Geometry check sheet. Reference: the model listing, model coordinates, mm. A direction names the side the tool comes from. Round coordinates to 2 decimals unless told otherwise and drop trailing zeros. Write each loop counter-clockwise with the first axis right and the second up, starting at its lowest first coordinate (ties: lowest second). Pieces come first, ordered by that corner, then holes. Notation, with made-up numbers: M 32,10 L 36,10 A22 ccw 36,41 Z; hole C 48,-11 d7. An arc over 180 degrees is marked long. One line per item, written item: value. Start each with the question number.
1. Section check C-C (x = 41). Record the boundary of the cut face in (y, z).
2. Depth check by flat-ended pin: P1, Ø5, axis at x = -25, z = -24, coming from the -Y side; P2, Ø1.5, axis at x = 97.5, z = 39.5, coming from the +Y side; P3, Ø0.6, axis at x = 139, z = 30, coming from the +Y side. Enter the tip coordinate at first touch or a pass-through.
3. Scan lines: probe 1 along Z at (x, y) = (125, -0.15); probe 2 along X at (y, z) = (8.5, 1); probe 3 along Z at (x, y) = (89, 10.25). Record each from-to range of solid material in increasing order. Write a range as [from, to].
4. Section check A-A (x = 125). Count the separate pieces of the cut face and the enclosed holes in it, and give its area (3 significant figures).
5. Access from +Z, -Z, +X, -X, +Y, -Y to the whole of each face (thin tool, end or side, straight path). Record for faces 1 (the cylindrical face through (120.786, -0.345, 0.553)), 2 (the flat face through (-71, 7, 71.3)), 3 (the flat face through (138.3, 6, 1)).
6. Release check for a two-part mould opening along X. For faces 4 (the flat face through (71, 7, -71.3)), 5 (the cylindrical face through (71.23, -0.35, 1.96)) record: pulls with the +X half, pulls with the -X half, needs draft (parallel to the pull), parting line crosses it, or undercut.
from build123d import *

# Parameters (mm, degrees)
SKETCH_1_W                         = 278
SKETCH_1_H                         = 144
SKETCH_1_R                         = 4.25
SM_BASE_FLANGE_1_DEPTH             = 0.7
SM_EDGE_FLANGE_1_STRIP_W           = 3.2
SM_EDGE_FLANGE_1_STRIP_H           = 0.7
SM_EDGE_FLANGE_1_STRIP_CUT_DEPTH   = 278
SM_EDGE_FLANGE_1_STRIP_2_W         = 3.2
SM_EDGE_FLANGE_1_STRIP_2_H         = 0.7
SM_EDGE_FLANGE_1_STRIP_CUT_2_DEPTH = 278
SM_EDGE_FLANGE_1_DEPTH             = 278
SM_EDGE_FLANGE_1_BEND_DEPTH        = 278
SKETCH_14_R                        = 3
CUT_EXTRUDE_1_DEPTH                = 10
SKETCH_15_R                        = 3
CUT_EXTRUDE_2_DEPTH                = 10
SKETCH_16_W                        = 3
SKETCH_16_H                        = 13.3
CUT_EXTRUDE_3_DEPTH                = 10
SKETCH_17_W                        = 3
SKETCH_17_H                        = 13.3
CUT_EXTRUDE_4_DEPTH                = 10
SM_EDGE_FLANGE_2_STRIP_W           = 3.2
SM_EDGE_FLANGE_2_STRIP_H           = 0.7
SM_EDGE_FLANGE_2_STRIP_CUT_DEPTH   = 142.2
SM_EDGE_FLANGE_2_STRIP_2_W         = 3.2
SM_EDGE_FLANGE_2_STRIP_2_H         = 0.7
SM_EDGE_FLANGE_2_STRIP_CUT_2_DEPTH = 142.2
SM_EDGE_FLANGE_2_DEPTH             = 142.2
SM_EDGE_FLANGE_2_BEND_DEPTH        = 142.2


# Sheet-metal steps are written as plain solids
with BuildPart() as part:
    # Sketch 1 → 基体-法兰1 (new body)
    with BuildSketch(Plane(origin=(0, 0, 0), x_dir=(1, 0, 0), z_dir=(0, 1, 0))):
        Rectangle(SKETCH_1_W, SKETCH_1_H)
        with Locations(Location((-125, -48, 0), (0, 0, 270))):
            Circle(SKETCH_1_R, mode=Mode.SUBTRACT)
        with Locations(Location((-125, -24, 0), (0, 0, 270))):
            Circle(SKETCH_1_R, mode=Mode.SUBTRACT)
        with Locations(Location((-125, 0, 0), (0, 0, 270))):
            Circle(SKETCH_1_R, mode=Mode.SUBTRACT)
        with Locations(Location((-125, 24, 0), (0, 0, 270))):
            Circle(SKETCH_1_R, mode=Mode.SUBTRACT)
        with Locations(Location((-125, 48, 0), (0, 0, 270))):
            Circle(SKETCH_1_R, mode=Mode.SUBTRACT)
        with Locations(Location((-75, -48, 0), (0, 0, 90))):
            Circle(SKETCH_1_R, mode=Mode.SUBTRACT)
        with Locations(Location((-75, -24, 0), (0, 0, 90))):
            Circle(SKETCH_1_R, mode=Mode.SUBTRACT)
        with Locations(Location((-75, 0, 0), (0, 0, 90))):
            Circle(SKETCH_1_R, mode=Mode.SUBTRACT)
        with Locations(Location((-75, 24, 0), (0, 0, 90))):
            Circle(SKETCH_1_R, mode=Mode.SUBTRACT)
        with Locations(Location((-75, 48, 0), (0, 0, 90))):
            Circle(SKETCH_1_R, mode=Mode.SUBTRACT)
        with Locations(Location((-25, -48, 0), (0, 0, 270))):
            Circle(SKETCH_1_R, mode=Mode.SUBTRACT)
        with Locations(Location((-25, -24, 0), (0, 0, 270))):
            Circle(SKETCH_1_R, mode=Mode.SUBTRACT)
        with Locations(Location((-25, 0, 0), (0, 0, 270))):
            Circle(SKETCH_1_R, mode=Mode.SUBTRACT)
        with Locations(Location((-25, 24, 0), (0, 0, 270))):
            Circle(SKETCH_1_R, mode=Mode.SUBTRACT)
        with Locations(Location((-25, 48, 0), (0, 0, 270))):
            Circle(SKETCH_1_R, mode=Mode.SUBTRACT)
        with Locations(Location((25, -48, 0), (0, 0, 90))):
            Circle(SKETCH_1_R, mode=Mode.SUBTRACT)
        with Locations(Location((25, -24, 0), (0, 0, 90))):
            Circle(SKETCH_1_R, mode=Mode.SUBTRACT)
        with Locations(Location((25, 0, 0), (0, 0, 90))):
            Circle(SKETCH_1_R, mode=Mode.SUBTRACT)
        with Locations(Location((25, 24, 0), (0, 0, 90))):
            Circle(SKETCH_1_R, mode=Mode.SUBTRACT)
        with Locations(Location((25, 48, 0), (0, 0, 90))):
            Circle(SKETCH_1_R, mode=Mode.SUBTRACT)
        with Locations(Location((75, 48, 0), (0, 0, 270))):
            Circle(SKETCH_1_R, mode=Mode.SUBTRACT)
        with Locations(Location((75, 24, 0), (0, 0, 270))):
            Circle(SKETCH_1_R, mode=Mode.SUBTRACT)
        with Locations(Location((75, 0, 0), (0, 0, 270))):
            Circle(SKETCH_1_R, mode=Mode.SUBTRACT)
        with Locations(Location((75, -24, 0), (0, 0, 270))):
            Circle(SKETCH_1_R, mode=Mode.SUBTRACT)
        with Locations(Location((75, -48, 0), (0, 0, 270))):
            Circle(SKETCH_1_R, mode=Mode.SUBTRACT)
        with Locations(Location((125, -48, 0), (0, 0, 90))):
            Circle(SKETCH_1_R, mode=Mode.SUBTRACT)
        with Locations(Location((125, -24, 0), (0, 0, 90))):
            Circle(SKETCH_1_R, mode=Mode.SUBTRACT)
        with Locations(Location((125, 0, 0), (0, 0, 90))):
            Circle(SKETCH_1_R, mode=Mode.SUBTRACT)
        with Locations(Location((125, 24, 0), (0, 0, 90))):
            Circle(SKETCH_1_R, mode=Mode.SUBTRACT)
        with Locations(Location((125, 48, 0), (0, 0, 90))):
            Circle(SKETCH_1_R, mode=Mode.SUBTRACT)
    extrude(amount=-SM_BASE_FLANGE_1_DEPTH)

    # 边线-法兰1 strip (across the edge) → 边线-法兰1 strip cut (cut)
    with BuildSketch(Plane(origin=(-139, 0, 72), x_dir=(0, 0, -1), z_dir=(1, 0, 0))):
        with Locations((-0.7, -0.35)):
            Rectangle(SM_EDGE_FLANGE_1_STRIP_W, SM_EDGE_FLANGE_1_STRIP_H)
    extrude(amount=SM_EDGE_FLANGE_1_STRIP_CUT_DEPTH, mode=Mode.SUBTRACT)

    # 边线-法兰1 strip 2 (across the edge) → 边线-法兰1 strip cut 2 (cut)
    with BuildSketch(Plane(origin=(139, 0, -72), x_dir=(0, 0, 1), z_dir=(-1, 0, 0))):
        with Locations((-0.7, -0.35)):
            Rectangle(SM_EDGE_FLANGE_1_STRIP_2_W, SM_EDGE_FLANGE_1_STRIP_2_H)
    extrude(amount=SM_EDGE_FLANGE_1_STRIP_CUT_2_DEPTH, mode=Mode.SUBTRACT)

    # 边线-法兰1 section (across the edge) → 边线-法兰1 (add)
    with BuildSketch(Plane(origin=(-139, 0, 72), x_dir=(0, 0, -1), z_dir=(1, 0, 0))):
        with BuildLine():
            Line((0, 0.2), (0, 13.3))
            Line((0, 13.3), (0.7, 13.3))
            Line((0.7, 13.3), (0.7, 0.2))
            ThreePointArc((0.7, 0.2), (0.758578644, 0.058578644), (0.9, 0))
            Line((0.9, 0), (0.9, -0.7))
            ThreePointArc((0.9, -0.7), (0.263603897, -0.436396103), (0, 0.2))
        make_face()
    extrude(amount=SM_EDGE_FLANGE_1_DEPTH)

    # 边线-法兰1 section 2 (across the edge) → 边线-法兰1 bend (add)
    with BuildSketch(Plane(origin=(139, 0, -72), x_dir=(0, 0, 1), z_dir=(-1, 0, 0))):
        with BuildLine():
            Line((0, 0.2), (0, 13.3))
            Line((0, 13.3), (0.7, 13.3))
            Line((0.7, 13.3), (0.7, 0.2))
            ThreePointArc((0.7, 0.2), (0.758578644, 0.058578644), (0.9, 0))
            Line((0.9, 0), (0.9, -0.7))
            ThreePointArc((0.9, -0.7), (0.263603897, -0.436396103), (0, 0.2))
        make_face()
    extrude(amount=SM_EDGE_FLANGE_1_BEND_DEPTH)

    # 草图14 → 切除-拉伸1 (cut)
    with BuildSketch(Plane(origin=(0, 0, 71.3), x_dir=(-1, 0, 0), z_dir=(0, 0, -1))):
        with Locations((-133.5, 7.8)):
            Circle(SKETCH_14_R)
        with Locations((0, 7.8)):
            Circle(SKETCH_14_R)
        with Locations((133.5, 7.8)):
            Circle(SKETCH_14_R)
    extrude(amount=-CUT_EXTRUDE_1_DEPTH, mode=Mode.SUBTRACT)

    # 草图15 → 切除-拉伸2 (cut)
    with BuildSketch(Plane(origin=(0, 0, -72), x_dir=(-1, 0, 0), z_dir=(0, 0, -1))):
        with Locations((-133.5, 7.8)):
            Circle(SKETCH_15_R)
        with Locations((0, 7.8)):
            Circle(SKETCH_15_R)
        with Locations((133.5, 7.8)):
            Circle(SKETCH_15_R)
    extrude(amount=-CUT_EXTRUDE_2_DEPTH, mode=Mode.SUBTRACT)

    # 草图16 → 切除-拉伸3 (cut)
    with BuildSketch(Plane(origin=(0, 0, -72), x_dir=(-1, 0, 0), z_dir=(0, 0, -1))):
        with Locations((0, 6.65)):
            Rectangle(SKETCH_16_W, SKETCH_16_H)
    extrude(amount=-CUT_EXTRUDE_3_DEPTH, mode=Mode.SUBTRACT)

    # 草图17 → 切除-拉伸4 (cut)
    with BuildSketch(Plane.XY.offset(72)):
        with Locations((0, 6.65)):
            Rectangle(SKETCH_17_W, SKETCH_17_H)
    extrude(amount=-CUT_EXTRUDE_4_DEPTH, mode=Mode.SUBTRACT)

    # 边线-法兰2 strip (across the edge) → 边线-法兰2 strip cut (cut)
    with BuildSketch(Plane(origin=(-139, 0, -71.1), x_dir=(1, 0, 0), z_dir=(0, 0, 1))):
        with Locations((-0.7, -0.35)):
            Rectangle(SM_EDGE_FLANGE_2_STRIP_W, SM_EDGE_FLANGE_2_STRIP_H)
    extrude(amount=SM_EDGE_FLANGE_2_STRIP_CUT_DEPTH, mode=Mode.SUBTRACT)

    # 边线-法兰2 strip 2 (across the edge) → 边线-法兰2 strip cut 2 (cut)
    with BuildSketch(Plane(origin=(139, 0, 71.1), x_dir=(-1, 0, 0), z_dir=(0, 0, -1))):
        with Locations((-0.7, -0.35)):
            Rectangle(SM_EDGE_FLANGE_2_STRIP_2_W, SM_EDGE_FLANGE_2_STRIP_2_H)
    extrude(amount=SM_EDGE_FLANGE_2_STRIP_CUT_2_DEPTH, mode=Mode.SUBTRACT)

    # 边线-法兰2 section (across the edge) → 边线-法兰2 (add)
    with BuildSketch(Plane(origin=(-139, 0, -71.1), x_dir=(1, 0, 0), z_dir=(0, 0, 1))):
        with BuildLine():
            Line((0, 0.2), (0, 11.8))
            Line((0, 11.8), (0.7, 11.8))
            Line((0.7, 11.8), (0.7, 0.2))
            ThreePointArc((0.7, 0.2), (0.758578644, 0.058578644), (0.9, 0))
            Line((0.9, 0), (0.9, -0.7))
            ThreePointArc((0.9, -0.7), (0.263603897, -0.436396103), (0, 0.2))
        make_face()
    extrude(amount=SM_EDGE_FLANGE_2_DEPTH)

    # 边线-法兰2 section 2 (across the edge) → 边线-法兰2 bend (add)
    with BuildSketch(Plane(origin=(139, 0, 71.1), x_dir=(-1, 0, 0), z_dir=(0, 0, -1))):
        with BuildLine():
            Line((0, 0.2), (0, 11.8))
            Line((0, 11.8), (0.7, 11.8))
            Line((0.7, 11.8), (0.7, 0.2))
            ThreePointArc((0.7, 0.2), (0.758578644, 0.058578644), (0.9, 0))
            Line((0.9, 0), (0.9, -0.7))
            ThreePointArc((0.9, -0.7), (0.263603897, -0.436396103), (0, 0.2))
        make_face()
    extrude(amount=SM_EDGE_FLANGE_2_BEND_DEPTH)


solid = part.part
Result sheet:
1. outline: M -0.7,-71.1 A0.9 ccw 0.2,-72 L 13.3,-72 L 13.3,-71.3 L 0.2,-71.3 A0.2 cw 0,-71.1 L 0,71.1 A0.2 cw 0.2,71.3 L 13.3,71.3 L 13.3,72 L 0.2,72 A0.9 ccw -0.7,71.1 Z
2. P1: passes through
2. P2: stops at y = 0
2. P3: stops at y = 11.8
3. probe 1: z = [-71.93, -52.25], [-43.75, -28.25], [-19.75, -4.25], [4.25, 19.75], [28.25, 43.75], [52.25, 71.93]
3. probe 2: x = [-139, -138.3], [138.3, 139]
3. probe 3: z = [-72, -71.3], [71.3, 72]
4. separate pieces: 6
4. enclosed holes: 0
4. area: 89.3 mm2
5. face 1: +Y, -Y
5. face 2: +X, -X, +Y
5. face 3: +Y
6. face 4: needs draft
6. face 5: undercut
